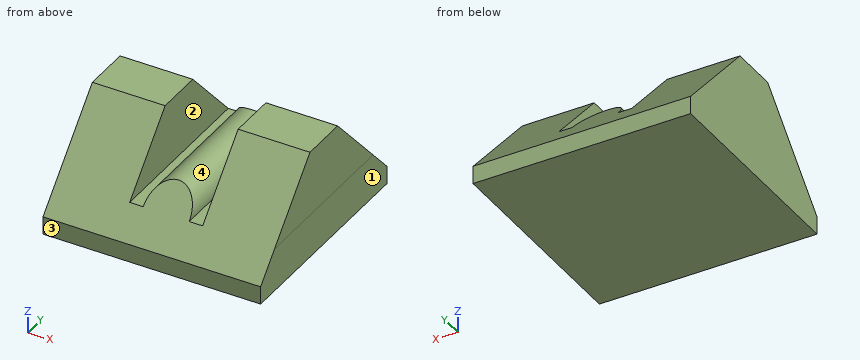
from build123d import *

# Parameters (mm, degrees)
F1_DEPTH = 25.4
F3_W     = 42.476376
F3_H     = 127
F4_DEPTH = 38.1
F2_W     = 41.917417
F2_H     = 127
F5_DEPTH = 38.1
F7_DEPTH = 127
F9_DEPTH = 127.001


with BuildPart() as f1:
    # F0 (on Top) → F1 (new body)
    with BuildSketch(Plane.XY):
        Polygon((63.5, 63.5), (0, 63.5), (-63.5, 63.5), (-63.5, 0), (-63.5, -63.5), (0, -63.5), (63.5, -63.5), (63.5, 0), align=None)
    extrude(amount=F1_DEPTH)

    # F3 (on face) → F4 (join)
    with BuildSketch(Plane.XY.offset(25.4)):
        with Locations((-42.261812, 0)):
            Rectangle(F3_W, F3_H)
    extrude(amount=F4_DEPTH)

    # F2 (on face) → F5 (join)
    with BuildSketch(Plane.XY.offset(25.4)):
        with Locations((42.541291, 0)):
            Rectangle(F2_W, F2_H)
    extrude(amount=F5_DEPTH)

    # F6 (on face) → F7 (join)
    with BuildSketch(Plane.XZ.offset(63.5)):
        with BuildLine():
            Line((-13.162336, 25.4), (13.721296, 25.4))
            ThreePointArc((13.721296, 25.4), (0.27948, 38.841816), (-13.162336, 25.4))
        make_face()
    extrude(amount=-F7_DEPTH)

    # F8 (on face) → F9 (cut, through all)
    with BuildSketch(Plane.YZ.offset(63.5)):
        Polygon((-63.5, 10.476396), (-13.906721, 63.5), (-63.5, 63.5), align=None)
        Polygon((63.5, 10.476396), (63.5, 63.5), (13.906721, 63.5), align=None)
    extrude(amount=-F9_DEPTH, mode=Mode.SUBTRACT)


solid = f1.part
Could you check a few things on this model? Use its own coordinates, in mm. Face numbers are marked on the shaded views. Give positions to 0.01 mm unless a question says otherwise; leave off trailing zeros. Order: outer loops, then holes, each group sorted by start corner. A loop starts at its lowest first (then second) coordinate and runs counter-clockwise, first axis right, second up.
1. I need wall thicknesses on L1, parallel to X at y = 17, z = 40.5; L2, parallel to X at y = 35, z = 27.5; L3, parallel to X at y = 30, z = 32. Which ranges of each line are inside material? Lowest first, please.
Answers below:
L1: x = -63.5 to -21.02, 21.58 to 63.5
L2: x = -63.5 to -21.02, -13 to 13.56, 21.58 to 63.5
L3: x = -63.5 to -21.02, -11.43 to 11.99, 21.58 to 63.5
2. For pin 1 (4 mm diameter, centred on x = -44, y = 4.5, fed in from -Z); pin 2 (5 mm diameter, centred on x = 30.5, y = 32.5, fed in from +Z); pin 3 (6.5 mm diameter, centred on x = -16.5, y = -16, fed in from +Z); pin 4 (12 mm diameter, centred on x = 49, y = -35.5, fed in from +Z), each with a flat end and sliding along its axis, tell me the tip position at first contact or that it passes through.
Answers below:
pin 1: stops at z = 0
pin 2: stops at z = 46.29
pin 3: stops at z = 25.4
pin 4: stops at z = 46.83
3. Thinking about a two-plate mould opening in X: for the marked faces 1, 2, 3 and 4, which applies, +X half, -X half, draft (parallel to the pull), parting line (faces both ways), or undercut?
Answers below:
face 1: +X half
face 2: undercut
face 3: draft
face 4: undercut
4. Suppose I cut it at C-C (y = -6). Write out the boundary of the cut face in (x, z), plus the area to 4 significant figures.
Answers below:
outline: (-63.5, 0) - (63.5, 0) - (63.5, 63.5) - (21.58, 63.5) - (21.58, 25.4) - (13.72, 25.4) arc R13.44 ccw to (-13.16, 25.4) - (-21.02, 25.4) - (-21.02, 63.5) - (-63.5, 63.5) - close
area: 6,725 mm2
5. Suppose I cut it at B-B (x = 54.5). Write out the boundary of the cut face in (y, z), plus the area to 3 significant figures.
Answers below:
outline: (-63.5, 0) - (63.5, 0) - (63.5, 10.48) - (13.91, 63.5) - (-13.91, 63.5) - (-63.5, 10.48) - close
area: 5,430 mm2
6. Suppose I cut it at D-D (z = 28.5). Write out the boundary of the cut face in (x, y).
Answers below:
outline: (-63.5, -46.64) - (-21.02, -46.64) - (-21.02, 46.64) - (-63.5, 46.64) - close; (-12.8, -46.64) - (13.36, -46.64) - (13.36, 46.64) - (-12.8, 46.64) - close; (21.58, -46.64) - (63.5, -46.64) - (63.5, 46.64) - (21.58, 46.64) - close
7. Suppose I cut it at A-A (z = 46). Write out the boundary of the cut face in (x, y).
Answers below:
outline: (-63.5, -30.27) - (-21.02, -30.27) - (-21.02, 30.27) - (-63.5, 30.27) - close; (21.58, -30.27) - (63.5, -30.27) - (63.5, 30.27) - (21.58, 30.27) - close
